The figure shows three views and two pictorial views of one solid part (mm, origin at its lowest corner). Answer the questions. A direction names the side the tool comes from. Coordinates: 2 decimals unless noted, no trailing zeros. Loops run counter-clockwise (first coordinate to the right, second up) from the corner with the lowest first, then second, coordinate; pieces in that order, holes last.
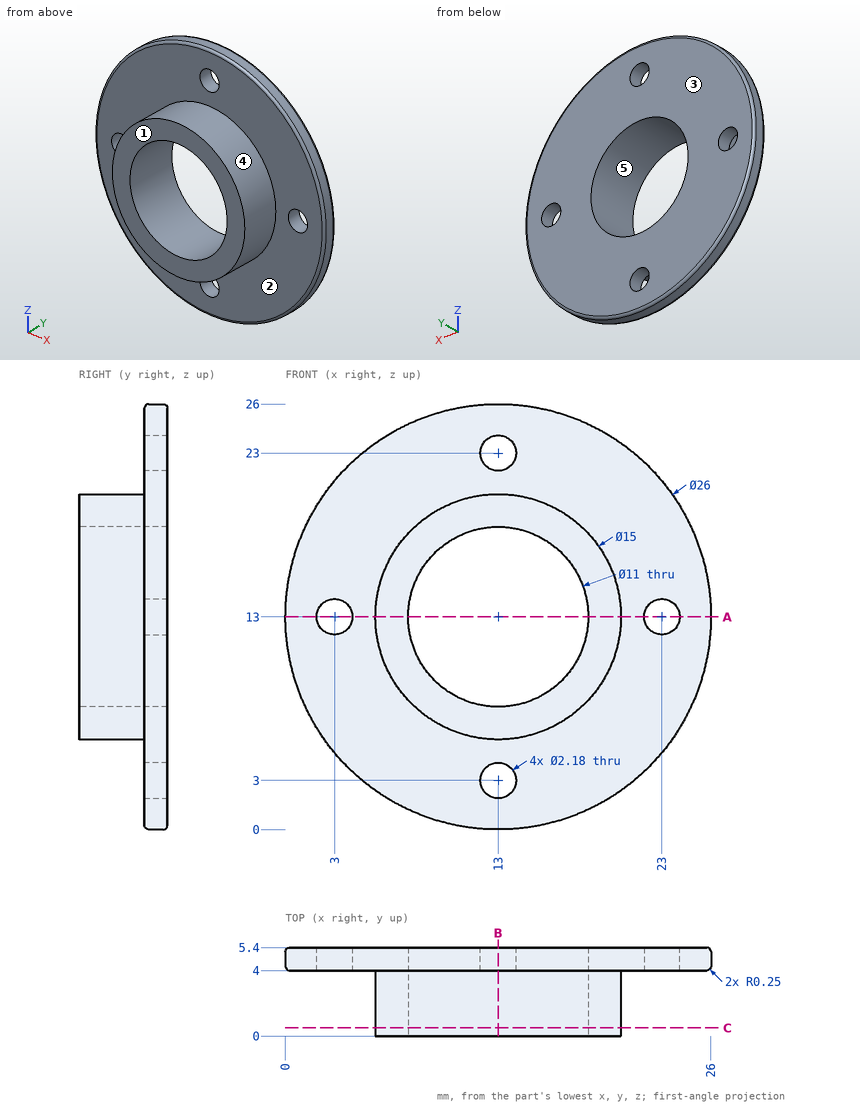
Q1. A cutting plane is placed at B-B (x = 13). Count the separate pieces of the cut face and the enclosed holes in it, then the cut area to 3 significant figures.
Findings below:
separate pieces: 4
enclosed holes: 0
area: 30.8 mm2
Q2. Straight lines are drawn through the part: probe 1 along Y at (x, z) = (8, 7); probe 2 along X at (y, z) = (2.3, 13); probe 3 along Z at (x, y) = (14.5, 1). For each, find the intervals that lie inside material, in ascending order.
Findings below:
probe 1: y = 4 to 5.4
probe 2: x = 5.5 to 7.5, 18.5 to 20.5
probe 3: z = 5.65 to 7.71, 18.29 to 20.35
Q3. Which of the six approach directions +Z, -Z, +X, -X, +Y, -Y give full straight-line access (tool end or side, diameter ignored) to the marked faces 1 and 2?
Findings below:
face 1: +Z, -Z, +X, -X, -Y
face 2: -Y
Q4. A cutting plane is placed at A-A (z = 13). Give the vertices of the cut face in (x, y).
Findings below:
outline: (0, 4.25) arc R0.25 ccw to (0.25, 4) - (1.91, 4) - (1.91, 5.4) - (0.25, 5.4) arc R0.25 ccw to (0, 5.15) - close; (4.09, 4) - (5.5, 4) - (5.5, 0) - (7.5, 0) - (7.5, 5.4) - (4.09, 5.4) - close; (18.5, 0) - (20.5, 0) - (20.5, 4) - (21.91, 4) - (21.91, 5.4) - (18.5, 5.4) - close; (24.09, 4) - (25.75, 4) arc R0.25 ccw to (26, 4.25) - (26, 5.15) arc R0.25 ccw to (25.75, 5.4) - (24.09, 5.4) - close
Q5. Flat-ended cylindrical pins translate along their axes: pin 1 Ø1.7 at (x, z) = (3, 13) entering from -Y; pin 2 Ø3 at (x, y) = (6, 3.5) entering from +Z. Find the tip coordinate at first contact, or state that the pin passes through.
Findings below:
pin 1: passes through
pin 2: stops at z = 24.69
Q6. Determine the mould class of the marked faces 3, 4 and 5 for opening direction Z: +Z half, -Z half, draft (parallel to the pull), parting line (faces both ways), or undercut.
Findings below:
face 3: draft
face 4: parting line
face 5: undercut
Q7. A cutting plane is placed at C-C (y = 0.5). Give the vertices of the cut face in (x, z).
Findings below:
outline: circle Ø15 at (13, 13); hole circle Ø11 at (13, 13)
